Check sheet for the modelled part. Datum: model origin and axes. Units: mm. A direction names the side the tool comes from. Round coordinates to 2 decimals unless told otherwise and drop trailing zeros. Loops run counter-clockwise (first coordinate to the right, second up) from the corner with the lowest first, then second, coordinate; pieces in that order, holes last. Notation, with made-up numbers: (80, 82.5) - (134, 82.5) arc R25 cw to (134, 107.5) - close; hole circle Ø6 at (10, -37). An arc over 180 degrees is marked (long way). Put each result on its own line as item: value. Start each with the question number.
```python
from build123d import *

# Parameters (mm, degrees)
SKETCH1_R                 = 6
SKETCH1_R_2               = 3
BOSS_EXTRUDE1_DEPTH       = 6.5
SKETCH1_3_R               = 3
BOSS_EXTRUDE2_DEPTH       = 22
SKETCH1_4_R               = 18.4
SKETCH1_4_R_2             = 15.5
SKETCH1_4_R_3             = 6
SKETCH1_4_R_4             = 3
BOSS_EXTRUDE3_DEPTH       = 20
BOSS_EXTRUDE4_START       = -57.15
SKETCH1_5_R               = 15.5
SKETCH1_5_R_2             = 6
SKETCH1_5_R_3             = 3
BOSS_EXTRUDE4_DEPTH       = 57.15
M3X0_5_TAPPED_HOLE1_D     = 2.5
M3X0_5_TAPPED_HOLE1_DEPTH = 4.675
M3X0_5_TAPPED_HOLE1_TIP   = 0.751075774
CUT_EXTRUDE1_DEPTH        = 1
CUT_EXTRUDE2_START        = -12
CUT_EXTRUDE2_DEPTH        = 12
CHAMFER1_SIZE             = 1


with BuildPart() as part:
    # Sketch1 → Boss-Extrude1 (new body)
    with BuildSketch(Plane(origin=(0, 0, 0), x_dir=(0, 0, -1), z_dir=(1, 0, 0))):
        with Locations(Location((0, -7, 0), (0, 0, 180))):
            Circle(SKETCH1_R)
        with Locations(Location((0, -7, 0), (0, 0, 180))):
            Circle(SKETCH1_R_2, mode=Mode.SUBTRACT)
    extrude(amount=BOSS_EXTRUDE1_DEPTH)

    # Sketch1_3 → Boss-Extrude2 (add)
    with BuildSketch(Plane(origin=(0, 0, 0), x_dir=(0, 0, -1), z_dir=(1, 0, 0))):
        with Locations((0, -7)):
            Circle(SKETCH1_3_R)
    extrude(amount=BOSS_EXTRUDE2_DEPTH)



with BuildPart() as body_2:
    # Sketch1_4 → Boss-Extrude3 (new body)
    # profile 1 of 4: a face of its own
    with BuildSketch(Plane(origin=(0, 0, 0), x_dir=(0, 0, -1), z_dir=(1, 0, 0))):
        Circle(SKETCH1_4_R)
        Circle(SKETCH1_4_R_2, mode=Mode.SUBTRACT)
    # profile 2 of 4: a face of its own
    with BuildSketch(Plane(origin=(0, 0, 0), x_dir=(0, 0, -1), z_dir=(1, 0, 0))):
        Circle(SKETCH1_4_R_2)
        with Locations(Location((0, -7, 0), (0, 0, 180))):
            Circle(SKETCH1_4_R_3, mode=Mode.SUBTRACT)
    # profile 3 of 4: a face of its own
    with BuildSketch(Plane(origin=(0, 0, 0), x_dir=(0, 0, -1), z_dir=(1, 0, 0))):
        with Locations(Location((0, -7, 0), (0, 0, 180))):
            Circle(SKETCH1_4_R_3)
        with Locations((0, -7)):
            Circle(SKETCH1_4_R_4, mode=Mode.SUBTRACT)
    # profile 4 of 4: a face of its own
    with BuildSketch(Plane(origin=(0, 0, 0), x_dir=(0, 0, -1), z_dir=(1, 0, 0))):
        with Locations((0, -7)):
            Circle(SKETCH1_4_R_4)
    extrude(amount=-BOSS_EXTRUDE3_DEPTH)


with BuildPart() as part_1:
    add(part.part)

    add(body_2.part)  # Boss-Extrude4 merges body 2
    # Sketch1_5 → Boss-Extrude4 (add)
    # profile 1 of 3: a face of its own
    with BuildSketch(Plane(origin=(0, 0, 0), x_dir=(0, 0, -1), z_dir=(1, 0, 0)).offset(BOSS_EXTRUDE4_START)):
        Circle(SKETCH1_5_R)
        with Locations(Location((0, -7, 0), (0, 0, 180))):
            Circle(SKETCH1_5_R_2, mode=Mode.SUBTRACT)
    # profile 2 of 3: a face of its own
    with BuildSketch(Plane(origin=(0, 0, 0), x_dir=(0, 0, -1), z_dir=(1, 0, 0)).offset(BOSS_EXTRUDE4_START)):
        with Locations(Location((0, -7, 0), (0, 0, 180))):
            Circle(SKETCH1_5_R_2)
        with Locations((0, -7)):
            Circle(SKETCH1_5_R_3, mode=Mode.SUBTRACT)
    # profile 3 of 3: a face of its own
    with BuildSketch(Plane(origin=(0, 0, 0), x_dir=(0, 0, -1), z_dir=(1, 0, 0)).offset(BOSS_EXTRUDE4_START)):
        with Locations((0, -7)):
            Circle(SKETCH1_5_R_3)
    extrude(amount=BOSS_EXTRUDE4_DEPTH)

    # M3x0.5 Tapped Hole1
    with Locations(Plane(origin=(0, 0, 0), x_dir=(0, 0, -1), z_dir=(1, 0, 0))):
        with Locations((-13.423393759, 7.75), (-15.5, 0), (-13.423393759, -7.75), (-7.75, -13.423393759), (0, -15.5), (7.75, -13.423393759), (13.423393759, -7.75), (15.5, 0), (13.423393759, 7.75), (7.75, 13.423393759), (0, 15.5), (-7.75, 13.423393759)):
            Hole(M3X0_5_TAPPED_HOLE1_D / 2, depth=M3X0_5_TAPPED_HOLE1_DEPTH)
            with Locations((0, 0, -(M3X0_5_TAPPED_HOLE1_DEPTH + M3X0_5_TAPPED_HOLE1_TIP / 2))):  # 118° drill point
                Cone(0, M3X0_5_TAPPED_HOLE1_D / 2, M3X0_5_TAPPED_HOLE1_TIP, mode=Mode.SUBTRACT)

    # Sketch4 → Cut-Extrude1 (cut)
    with BuildSketch(Plane(origin=(0, 0, 0), x_dir=(0, 0, -1), z_dir=(1, 0, 0))):
        with BuildLine():
            ThreePointArc((11.347397534, -4.615091463), (0, 12.25), (-11.347397534, -4.615091463))
            ThreePointArc((-11.347397534, -4.615091463), (-9.427730891, -5.860483562), (-7.595808961, -4.489285714))
            ThreePointArc((-7.595808961, -4.489285714), (0, 1), (7.595808961, -4.489285714))
            ThreePointArc((7.595808961, -4.489285714), (9.427730891, -5.860483562), (11.347397534, -4.615091463))
        make_face()
    extrude(amount=-CUT_EXTRUDE1_DEPTH, mode=Mode.SUBTRACT)

    # Sketch5 → Cut-Extrude2 (cut)
    with BuildSketch(Plane(origin=(22, 0, 0), x_dir=(0, 0, -1), z_dir=(1, 0, 0)).offset(CUT_EXTRUDE2_START)):
        with BuildLine():
            Line((-1.8, -4.6), (1.8, -4.6))
            ThreePointArc((1.8, -4.6), (0, -4), (-1.8, -4.6))
        make_face()
    extrude(amount=CUT_EXTRUDE2_DEPTH, mode=Mode.SUBTRACT)

    # Chamfer1
    chamfer1_edges = [part_1.edges().sort_by_distance(p)[0] for p in [
        (6.5, -7, -6),
    ]]
    chamfer(chamfer1_edges, length=CHAMFER1_SIZE)


solid = part_1.part
```
Q1. Cross-section at C-C on y = 4.5. Enter the section's corners in (x, z).
Q2. Depth check by flat-ended pin: pin 1 Ø1.5 at (x, z) = (-39.5, -6) entering from -Y; pin 2 Ø12 at (y, z) = (-8.5, -9) entering from +X; pin 3 Ø3 at (x, z) = (-12.5, -7) entering from +Y. Enter the tip coordinate at first touch or a pass-through.
Q3. Cross-section at B-B on x = -37. Enter the section's corners in (y, z).
Q4. Set-up check for faces 5 (the face through (-2.37, 0.05, -16.75)), 6 (the face through (-9.9, -11.2, 14.6)), 7 (the face through (16, -4.6, 0)): record each of +Z, -Z, +X, -X, +Y, -Y from which the full face is reachable in a straight line by a thin tool's end or side.
Q5. Draft check along Y on faces 1 (the face through (-38.835, 15.368, 2.018)), 2 (the face through (-2.37, -8.97, 13.15)), 3 (the face through (6.5, -7.1, 3.3)), 4 (the face through (-5.296, 7.897, -13.263)). Enter one of: +Y half, -Y half, draft (parallel to the pull), parting line (faces both ways), or undercut.
Q6. Material ranges on line 1 (Y direction, x = -4.5, z = 8); line 2 (Z direction, x = -2, y = 7); line 3 (Y direction, x = -38, z = 5), recorded low to high. Write a range as from..to.
Q7. Cross-section at D-D on x = -9. Enter the section's corners in (y, z), and give its area (3 significant figures).
Q8. Cross-section at A-A on z = -10.5. Enter the section's corners in (x, y).
Answer list:
1. outline: (-57.15, -14.83) - (-20, -14.83) - (-20, -17.84) - (0, -17.84) - (0, -11.39) - (-1, -11.39) - (-1, 11.39) - (0, 11.39) - (0, 17.84) - (-20, 17.84) - (-20, 14.83) - (-57.15, 14.83) - close
2. pin 1: stops at y = -14.58
2. pin 2: stops at x = 6.5
2. pin 3: stops at y = 17.56
3. outline: circle Ø31 at (0, 0)
4. face 5: +X
4. face 6: +X, -X
4. face 7: +Z, -Z, +X, +Y
5. face 1: parting line
5. face 2: undercut
5. face 3: draft
5. face 4: undercut
6. line 1: y = -16.57..-14.65, -12.2..12.2, 14.65..16.57
6. line 2: z = -17.02..-14.42, -12.42..12.42, 14.42..17.02
6. line 3: y = -14.67..14.67
7. outline: circle Ø36.8 at (0, 0)
7. area: 1,060 mm2
8. outline: (-57.15, -11.4) - (-20, -11.4) - (-20, -15.11) - (0, -15.11) - (0, -5.59) - (-1, -5.59) - (-1, 6.31) - (0, 6.31) - (0, 15.11) - (-20, 15.11) - (-20, 11.4) - (-57.15, 11.4) - close
